Autodesk Inventor part; units mm, degrees
ref_plane "YZ Plane" through (0, 0, 0) normal (1, 0, 0) x (0, 1, 0)
ref_plane "XZ Plane" through (0, 0, 0) normal (0, 1, 0) x (-1, 0, 0)
ref_plane "XY Plane" through (0, 0, 0) normal (0, 0, 1) x (1, 0, 0)
sketch "Sketch1" plane through (0, 0, 0) normal (0, 0, 1) x (1, 0, 0)
  line L0 (15, 0) -> (125, 0)
  line L1 (140, 15) -> (140, 115)
  line L2 (125, 130) -> (15, 130)
  line L3 (0, 115) -> (0, 15)
  arc A0 (15, 130) -> (0, 115) centre (15, 115) ccw
  arc A1 (140, 115) -> (125, 130) centre (125, 115) ccw
  arc A2 (125, 0) -> (140, 15) centre (125, 15) ccw
  arc A3 (0, 15) -> (15, 0) centre (15, 15) ccw
  circle A4 centre (15, 115) radius 2
  circle A5 centre (125, 115) radius 2
  circle A6 centre (15, 15) radius 2
  circle A7 centre (125, 15) radius 2
  line L4 (61, 17.5) -> (79, 17.5) construction
  line L5 (79, 17.5) -> (79, 26.5) construction
  line L6 (79, 26.5) -> (61, 26.5) construction
  line L7 (61, 26.5) -> (61, 17.5) construction
  line L8 (61, 17.5) -> (79, 26.5) construction
  line L9 (79, 17.5) -> (61, 26.5) construction
  line L10 (70, 0) -> (70, 130) construction
  circle A8 centre (61, 26.5) radius 2
  circle A9 centre (61, 17.5) radius 2
  circle A10 centre (79, 26.5) radius 2
  circle A11 centre (79, 17.5) radius 2
  point P0 (0, 0)
  point P1 (140, 130)
  point P2 (140, 0)
  point P3 (0, 130)
  point P4 (70, 22)
  point P5 (70, 17.5)
  dimension "d0" = 140
  dimension "d1" = 130
  dimension "d2" = 15
  dimension "d3" = 4
  dimension "d4" = 4
  dimension "d5" = 4
  dimension "d6" = 4
  dimension "d7" = 18
  dimension "d8" = 9
  dimension "d9" = 17.5
  dimension "d11" = 4
  dimension "d12" = 4
extrude "Extrusion1" add sketch "Sketch1" along normal blind 3.7
properties part number "Base" material "PMMA Plastic"
Source: CAD feature listing. Evaluate the final solid. Frame: model axes, mm. Coordinates: 2 decimals unless noted, no trailing zeros. Loops run counter-clockwise (first coordinate to the right, second up) from the corner with the lowest first, then second, coordinate; pieces in that order, holes last. Notation, with made-up numbers: (87, 18.5) - (106, 18.5) arc R22 ccw to (106, 41.5) - close; hole circle Ø2 at (43, -6.5). An arc over 180 degrees is marked (long way). Return JSON: item names as keys, results as strings.
Q1. Material intervals for line 1 along Y through (x, z) = (61, 1.25); line 2 along Y through (x, z) = (59.5, 1.15); line 3 along Y through (x, z) = (129, 2.6), sorted ascending.
Results:
{"line 1": "0 to 15.5, 19.5 to 24.5, 28.5 to 130", "line 2": "0 to 16.18, 18.82 to 25.18, 27.82 to 130", "line 3": "0.54 to 129.46"}
Q2. Section C-C, the plane x = 130.5. Return loops of the section in (y, z), plus the area to 3 significant figures.
Results:
{"outline": "(1.04, 0) - (128.96, 0) - (128.96, 3.7) - (1.04, 3.7) - close", "area": "473 mm2"}
Q3. Mould query, pull axis X, two halves, no side actions, for faces 1 (the cylindrical face through (80.847, 27.266, 1.824)), 2 (the cylindrical face through (135.72, 4.51, 1.82)), 3 (the cylindrical face through (123.526, 113.648, 1.824)), 4 (the flat face through (69, 0, 2)). Classes: released by +X, released by -X, zero draft, split by the parting line, or undercut.
Results:
{"face 1": "undercut", "face 2": "released by +X", "face 3": "undercut", "face 4": "zero draft"}
Q4. Section B-B, the plane z = 2.5. Give the number of separate pieces and of enclosed holes in the cut face, plus the area to 3 significant figures.
Results:
{"separate pieces": "1", "enclosed holes": "8", "area": "17,900 mm2"}
Q5. Contact query for flat-ended pins moving along their axis: P1, Ø6.5, axis at x = 125, y = 15, coming from the -Z side; P2, Ø2.5, axis at x = 61, y = 17.5, coming from the -Z side. Output: stop coordinate, or through.
Results:
{"P1": "z = 0", "P2": "through"}
Q6. Section A-A, the plane x = 79. Return loops of the section in (y, z).
Results:
{"outline": "(0, 0) - (15.5, 0) - (15.5, 3.7) - (0, 3.7) - close; (19.5, 0) - (24.5, 0) - (24.5, 3.7) - (19.5, 3.7) - close; (28.5, 0) - (130, 0) - (130, 3.7) - (28.5, 3.7) - close"}
